Geometry check sheet. Reference: the model listing, model coordinates, mm. A direction names the side the tool comes from. Coordinates: 2 decimals unless noted, no trailing zeros. Order: outer loops, then holes, each group sorted by start corner. A loop starts at its lowest first (then second) coordinate and runs counter-clockwise, first axis right, second up. Notation, with made-up numbers: M 80.25,39.25 L 134.25,39.25 A6 cw 134.25,48.25 Z; hole C 33,5.5 d1. An arc over 180 degrees is marked long. One line per item, written item: value. Start each with the question number.
1) Sectioned sample at B-B, the plane y = 6.5. Enter the section's corners in (x, z), then the cut area to 3 significant figures.
2) Go/stop test with a flat-tipped pin: P1, Ø3, axis at x = -12.5, y = -16.5, coming from the -Z side. Record where the tip stops, or that it passes through.
3) Sectioned sample at A-A, the plane z = -4.75. Enter the section's corners in (x, y).
4) Draft check along X on faces 1 (the flat face through (-10.14, -17.24, 4.93)), 2 (the flat face through (0, 0, 10)), 3 (the cylindrical face through (-0.54, -2.44, -7.4)). Enter one of: pulls with the +X half, pulls with the -X half, needs draft (parallel to the pull), parting line crosses it, or undercut.
5) Sectioned sample at D-D, the plane y = 0. Enter the section's corners in (x, z).
6) Thickness scan on L1, parallel to Y at x = 0, z = -5; L2, parallel to Z at x = -2, y = 7.5; L3, parallel to Y at x = -2, z = -6. Record the ranges inside material, lowest first. Write a range as from..to.
7) Access from +Z, -Z, +X, -X, +Y, -Y to the whole of each face (thin tool, end or side, straight path). Record for faces 4 (the flat face through (9.86, -17.4, 4.93)), 5 (the cylindrical face through (-7.493, 0.33, -7.395)).
8) Sectioned sample at C-C, the plane x = 5. Enter the section's corners in (y, z).
```python
from build123d import *

# Parameters (mm, degrees)
SKETCH_R     = 7.5
SKETCH_R_2   = 2.5
PAD_DEPTH    = 15
PAD001_DEPTH = 10


with BuildPart() as part:
    # Sketch → Pad (new body)
    with BuildSketch(Plane.XY):
        Circle(SKETCH_R)
        Circle(SKETCH_R_2, mode=Mode.SUBTRACT)
    extrude(amount=-PAD_DEPTH)

    # Sketch001 → Pad001 (join)
    with BuildSketch(Plane.XY):
        Polygon((20, 11.547005), (0, 23.094011), (-20, 11.547005), (-20, -11.547005), (0, -23.094011), (20, -11.547005), align=None)
    extrude(amount=PAD001_DEPTH)


solid = part.part
```
Final values:
1. outline: M -20,0 L -3.74,0 L -3.74,-15 L 3.74,-15 L 3.74,0 L 20,0 L 20,10 L -20,10 Z
1. area: 512 mm^2
2. P1: stops at z = 0
3. outline: C 0,0 d15; hole C 0,0 d5
4. face 1: pulls with the -X half
4. face 2: needs draft
4. face 3: undercut
5. outline: M -20,0 L -7.5,0 L -7.5,-15 L -2.5,-15 L -2.5,0 L 2.5,0 L 2.5,-15 L 7.5,-15 L 7.5,0 L 20,0 L 20,10 L -20,10 Z
6. L1: y = -7.5..-2.5, 2.5..7.5
6. L2: z = 0..10
6. L3: y = -7.23..-1.5, 1.5..7.23
7. face 4: +Z, -Z, +X, -Y
7. face 5: -Z
8. outline: M -20.21,0 L -5.59,0 L -5.59,-15 L 5.59,-15 L 5.59,0 L 20.21,0 L 20.21,10 L -20.21,10 Z
